The figure shows three views and two pictorial views of one solid part (mm, origin at its lowest corner). Answer the questions. Round coordinates to 2 decimals unless told otherwise and drop trailing zeros. Order: outer loops, then holes, each group sorted by start corner. A loop starts at its lowest first (then second) coordinate and runs counter-clockwise, first axis right, second up. Notation, with made-up numbers: M 25.5,51 L 31.5,51 A24 ccw 31.5,71 Z; hole C 13,23 d9. An arc over 180 degrees is marked long. Answer as CSV lines item,"result".
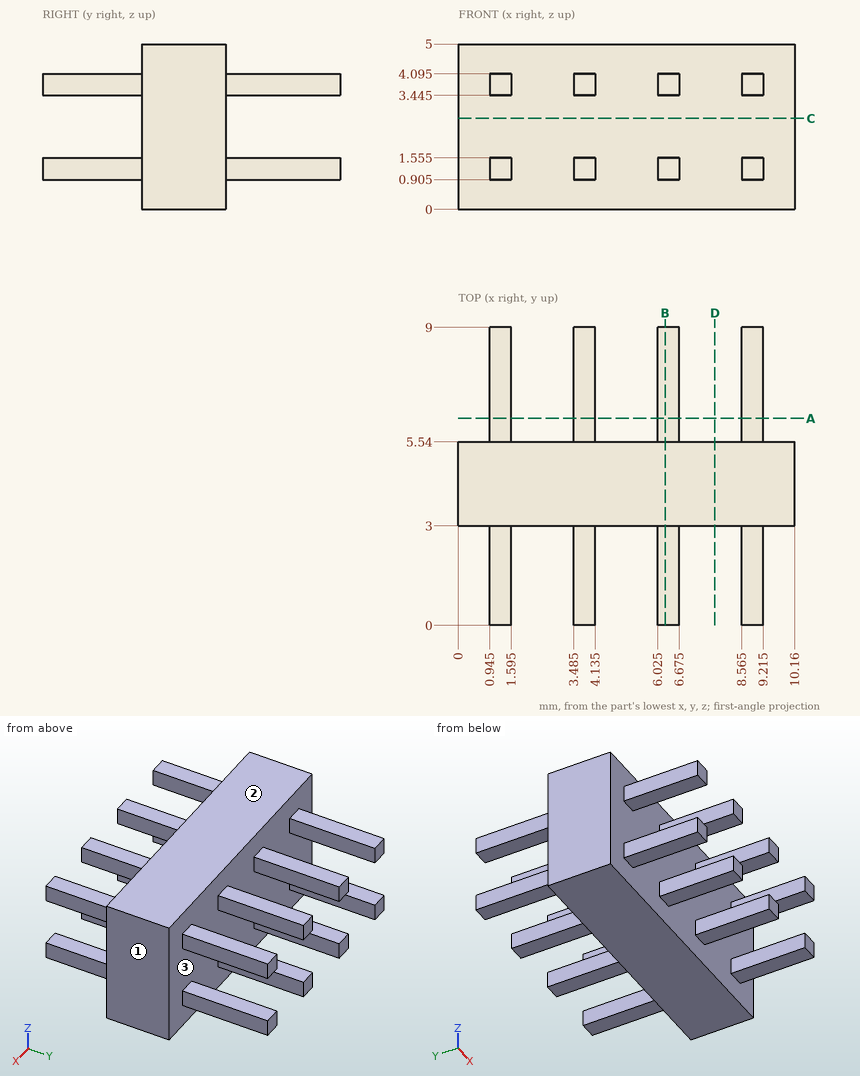
Item 1: A cutting plane is placed at B-B, the plane x = 6.25. Determine the outline of the cut face in (y, z) (3 decimals).
Ans:
outline,"M 0,0.905 L 3,0.905 L 3,0 L 5.54,0 L 5.54,0.905 L 9,0.905 L 9,1.555 L 5.54,1.555 L 5.54,3.445 L 9,3.445 L 9,4.095 L 5.54,4.095 L 5.54,5 L 3,5 L 3,4.095 L 0,4.095 L 0,3.445 L 3,3.445 L 3,1.555 L 0,1.555 Z"
Item 2: Find the intervals of material crossed by probe 1 along X at (y, z) = (8, 3.55) (3 decimals); probe 2 along Z at (x, y) = (8.75, 8.75) (3 decimals); probe 3 along Y at (x, z) = (6.5, 3.4), in increasing order. Write a range as [from, to].
Ans:
probe 1,"[0.945, 1.595], [3.485, 4.135], [6.025, 6.675], [8.565, 9.215]"
probe 2,"[0.905, 1.555], [3.445, 4.095]"
probe 3,"[3, 5.54]"
Item 3: A cutting plane is placed at A-A, the plane y = 6.25. Give the number of separate pieces and of enclosed holes in the cut face, and give its area (3 significant figures).
Ans:
separate pieces,"8"
enclosed holes,"0"
area,"3.38 mm2"
Item 4: A cutting plane is placed at C-C, the plane z = 2.75. Determine the outline of the cut face in (x, y), and give its area (3 significant figures).
Ans:
outline,"M 0,3 L 10.16,3 L 10.16,5.54 L 0,5.54 Z"
area,"25.8 mm2"
Item 5: Flat-ended cylindrical pins translate along their axes: pin 1 (0.7 mm diameter, centred on x = 9, y = 1.5, fed in from -Z) (3 decimals); pin 2 (0.7 mm diameter, centred on y = 7.5, z = 1.5, fed in from +X) (3 decimals); pin 3 (0.7 mm diameter, centred on x = 6.5, y = 2, fed in from +Z) (3 decimals). Find the tip coordinate at first contact, or state that the pin passes through.
Ans:
pin 1,"z = 0.905"
pin 2,"x = 9.215"
pin 3,"z = 4.095"
Item 6: Determine the mould class of the marked faces 1, 2 and 3 for opening direction X: +X half, -X half, draft (parallel to the pull), parting line (faces both ways), or undercut.
Ans:
face 1,"+X half"
face 2,"draft"
face 3,"undercut"
Item 7: A cutting plane is placed at D-D, the plane x = 7.75. Determine the outline of the cut face in (y, z).
Ans:
outline,"M 3,0 L 5.54,0 L 5.54,5 L 3,5 Z"
